Work out the finished part from the listing and answer in its coordinate system (mm). A direction names the side the tool comes from. Round coordinates to 2 decimals unless told otherwise and drop trailing zeros. Order: outer loops, then holes, each group sorted by start corner. A loop starts at its lowest first (then second) coordinate and runs counter-clockwise, first axis right, second up. Notation, with made-up numbers: (19, -21.5) -> (30, -21.5) arc R29 ccw to (30, 0.5) -> close; hole circle Ø10 at (-14.5, 67). An arc over 180 degrees is marked (long way). Use a Markdown table: item, result. Add a question column.
Item 1: A cutting plane is placed at C-C, the plane y = 27.75. Determine the outline of the cut face in (x, z), plus the area to 3 significant figures.
Item 2: A cutting plane is placed at B-B, the plane y = 14. Determine the outline of the cut face in (x, z), plus the area to 4 significant figures.
Item 3: A cutting plane is placed at D-D, the plane x = 50.5. Determine the outline of the cut face in (y, z).
Item 4: For a pull along Z with two mould halves and no side action, classify faces 1 (the cylindrical face through (67.966, 41.365, 1.726)), 2 (the flat face through (-2.3, 29.5, 7)), 3 (the cylindrical face through (62.081, -8.229, 12.974)) as +Z half, -Z half, draft (parallel to the pull), parting line (faces both ways), or undercut.
Item 5: Find the intervals of material crossed by L1, parallel to Y at x = 33, z = 3; L2, parallel to X at y = -9, z = 13.5; L3, parallel to X at y = 20.5, z = 2, in increasing order. Write a range as [from, to].
Item 6: Flat-ended cylindrical pins translate along their axes: P1, Ø0.9, axis at x = 34.5, y = -8.5, coming from the +Z side; P2, Ø1, axis at x = 73, z = 5.5, coming from the +Y side; P3, Ø10, axis at y = 1.5, z = 9.5, coming from the +X side; P4, Ø4, axis at x = -1.75, y = 27.75, coming from the +Z side. Find the tip coordinate at first contact, or state that the pin passes through.
Item 7: A tool of negligible diameter and unlimited length cuts with its end or side. For faces 4 (the flat face through (70.75, 28, 5)), 5 (the flat face through (23.75, -8, 13)), 6 (the flat face through (13.75, 39, 2)), from which of +Z, -Z, +X, -X, +Y, -Y can it reach the whole face along a straight path? Write none if from no direction.
Item 8: A cutting plane is placed at A-A, the plane x = 63.75. Determine the outline of the cut face in (y, z).
from build123d import *

# Parameters (mm, degrees)
SKETCH1_W           = 80
SKETCH1_H           = 36
SKETCH1_R           = 1.65
SKETCH1_W_2         = 71.5
SKETCH1_H_2         = 24.5
BOSS_EXTRUDE1_DEPTH = 3.5
SKETCH2_W           = 5
SKETCH2_H           = 5
SKETCH2_R           = 1.65
BOSS_EXTRUDE2_DEPTH = 3.5
BOSS_EXTRUDE4_DEPTH = 1
BOSS_EXTRUDE5_START = 1
SKETCH3_R           = 1.75
BOSS_EXTRUDE5_DEPTH = 3
SKETCH7_W           = 18
SKETCH7_H           = 18
SKETCH7_R           = 1.65
BOSS_EXTRUDE6_DEPTH = 3.5


with BuildPart() as part:
    # Sketch1 → Boss-Extrude1 (new body)
    with BuildSketch(Plane.XY):
        with Locations((35.75, 12.25)):
            Rectangle(SKETCH1_W, SKETCH1_H)
        with Locations((-1.75, 27.75)):
            Circle(SKETCH1_R, mode=Mode.SUBTRACT)
        with Locations((73.25, 27.75)):
            Circle(SKETCH1_R, mode=Mode.SUBTRACT)
        with Locations((73.25, -3.25)):
            Circle(SKETCH1_R, mode=Mode.SUBTRACT)
        with Locations((-1.75, -3.25)):
            Circle(SKETCH1_R, mode=Mode.SUBTRACT)
        with Locations((35.75, 12.25)):
            Rectangle(SKETCH1_W_2, SKETCH1_H_2, mode=Mode.SUBTRACT)
    extrude(amount=BOSS_EXTRUDE1_DEPTH)

    # Sketch2 → Boss-Extrude2 (add)
    with BuildSketch(Plane.XY.offset(3.5)):
        with Locations((-1.75, 27.75)):
            Rectangle(SKETCH2_W, SKETCH2_H)
        with Locations((-1.75, 27.75)):
            Circle(SKETCH2_R, mode=Mode.SUBTRACT)
        with Locations((73.25, 27.75)):
            Rectangle(SKETCH2_W, SKETCH2_H)
        with Locations((73.25, 27.75)):
            Circle(SKETCH2_R, mode=Mode.SUBTRACT)
        with Locations((-1.75, -3.25)):
            Rectangle(SKETCH2_W, SKETCH2_H)
        with Locations((-1.75, -3.25)):
            Circle(SKETCH2_R, mode=Mode.SUBTRACT)
        with Locations((73.25, -3.25)):
            Rectangle(SKETCH2_W, SKETCH2_H)
        with Locations((73.25, -3.25)):
            Circle(SKETCH2_R, mode=Mode.SUBTRACT)
    extrude(amount=BOSS_EXTRUDE2_DEPTH)

    # Sketch6 → Boss-Extrude4 (add)
    with BuildSketch(Plane.XZ.offset(5.75)):
        Polygon((-4.25, 0), (-4.25, 7), (0.75, 7), (0.75, 3.5), (70.75, 3.5), (70.75, 7), (75.75, 7), (75.75, 0), align=None)
    extrude(amount=BOSS_EXTRUDE4_DEPTH)

    # Sketch3 → Boss-Extrude5 (add)
    with BuildSketch(Plane(origin=(0, -5.75, 0), x_dir=(-1, 0, 0), z_dir=(0, -1, 0)).offset(BOSS_EXTRUDE5_START)):
        Polygon((-47.75, -17), (-47.75, -10), (-23.75, -10), (-23.75, -17), (4.25, -17), (4.25, 0), (-75.75, 0), (-75.75, -17), align=None)
        with Locations((-7.75, -13.5)):
            Circle(SKETCH3_R, mode=Mode.SUBTRACT)
        with Locations((-63.75, -13.5)):
            Circle(SKETCH3_R, mode=Mode.SUBTRACT)
    extrude(amount=BOSS_EXTRUDE5_DEPTH)

    # Sketch7 → Boss-Extrude6 (add)
    with BuildSketch(Plane(origin=(0, 0, 0), x_dir=(-1, 0, 0), z_dir=(0, 0, -1))):
        with Locations((-66.75, 39.25)):
            Rectangle(SKETCH7_W, SKETCH7_H)
        with Locations((-66.75, 40.25)):
            Circle(SKETCH7_R, mode=Mode.SUBTRACT)
        with Locations((-4.75, 39.25)):
            Rectangle(SKETCH7_W, SKETCH7_H)
        with Locations((-4.75, 40.25)):
            Circle(SKETCH7_R, mode=Mode.SUBTRACT)
    extrude(amount=-BOSS_EXTRUDE6_DEPTH)


solid = part.part
Reported:
| question | item | result |
|---|---|---|
| 1 | outline | (-4.25, 0) -> (-3.4, 0) -> (-3.4, 7) -> (-4.25, 7) -> close; (-0.1, 0) -> (71.6, 0) -> (71.6, 7) -> (70.75, 7) -> (70.75, 3.5) -> (0.75, 3.5) -> (0.75, 7) -> (-0.1, 7) -> close; (74.9, 0) -> (75.75, 0) -> (75.75, 7) -> (74.9, 7) -> close |
| 1 | area | 269 mm² |
| 2 | outline | (-4.25, 0) -> (0, 0) -> (0, 3.5) -> (-4.25, 3.5) -> close; (71.5, 0) -> (75.75, 0) -> (75.75, 3.5) -> (71.5, 3.5) -> close |
| 2 | area | 29.75 mm² |
| 3 | outline | (-9.75, 0) -> (0, 0) -> (0, 3.5) -> (-6.75, 3.5) -> (-6.75, 17) -> (-9.75, 17) -> close; (24.5, 0) -> (30.25, 0) -> (30.25, 3.5) -> (24.5, 3.5) -> close |
| 4 | face 1 | draft |
| 4 | face 2 | +Z half |
| 4 | face 3 | undercut |
| 5 | L1 | [-9.75, 0], [24.5, 30.25] |
| 5 | L2 | [-4.25, 6], [9.5, 23.75], [47.75, 62], [65.5, 75.75] |
| 5 | L3 | [-4.25, 0], [71.5, 75.75] |
| 6 | P1 | z = 10 |
| 6 | P2 | y = 30.25 |
| 6 | P3 | x = 75.75 |
| 6 | P4 | z = 7 |
| 7 | face 4 | +Z, +Y |
| 7 | face 5 | +Z, +Y, -Y |
| 7 | face 6 | +Z, -Z, +Y |
| 8 | outline | (-9.75, 0) -> (0, 0) -> (0, 3.5) -> (-6.75, 3.5) -> (-6.75, 11.75) -> (-9.75, 11.75) -> close; (-9.75, 15.25) -> (-6.75, 15.25) -> (-6.75, 17) -> (-9.75, 17) -> close; (24.5, 0) -> (48.25, 0) -> (48.25, 3.5) -> (24.5, 3.5) -> close |
